```python
from build123d import *

# Parameters (mm, degrees)
BASPROSKE_W         = 5
BASPROSKE_H         = 10
TOOTHCUT_DEPTH      = 16
TEETHCUTS_COUNT     = 18
TEETHCUTS_ANGLE     = 340
BORSKE_R            = 4
BORE_DEPTH          = 50.0000508
CUT_EXTRUDE_1_DEPTH = 2.5


with BuildPart() as part:
    # BasProSke → Base-Revolve (revolve)
    with BuildSketch(Plane(origin=(0, 0, 0), x_dir=(1, 0, 0), z_dir=(0, 1, 0)), mode=Mode.PRIVATE) as base_revolve_sk:
        with Locations((2.5, 5)):
            Rectangle(BASPROSKE_W, BASPROSKE_H)
    revolve(base_revolve_sk.sketch.rotate(Axis((-10, 0, 0), (1, 0, 0)), 180), axis=Axis((-10, 0, 0), (1, 0, 0)))

    # TooCutSke → ToothCut (cut, through all)
    with BuildSketch(Plane(origin=(0, 0, 0), x_dir=(0, 0, -1), z_dir=(1, 0, 0))):
        with BuildLine():
            ThreePointArc((0.510641536, 7.732156635), (0, 7.749), (-0.510641536, 7.732156635))
            ThreePointArc((-0.510641536, 7.732156635), (-0.82619259, 8.907320741), (-1.515208602, 9.910236529))
            ThreePointArc((-1.515208602, 9.910236529), (0, 10.0254), (1.515208602, 9.910236529))
            ThreePointArc((1.515208602, 9.910236529), (0.82619259, 8.907320741), (0.510641536, 7.732156635))
        make_face()
    toothcut = extrude(amount=TOOTHCUT_DEPTH, mode=Mode.SUBTRACT)

    # TeethCuts: ToothCut ×18 about axis
    teethcuts_axis = Axis((-10, 0, 0), (1, 0, 0))
    for i in range(1, TEETHCUTS_COUNT):
        add(toothcut.rotate(teethcuts_axis, i * TEETHCUTS_ANGLE / (TEETHCUTS_COUNT - 1)), mode=Mode.SUBTRACT)

    # BorSke → Bore (cut, symmetric)
    with BuildSketch(Plane(origin=(0, 0, 0), x_dir=(0, 0, -1), z_dir=(1, 0, 0))):
        with Locations(Location((0, 0, 0), (0, 0, 180))):
            Circle(BORSKE_R)
    extrude(amount=BORE_DEPTH, both=True, mode=Mode.SUBTRACT)

    # 草图2 → 切除-拉伸1 (cut)
    with BuildSketch(Plane.ZY):
        Polygon((0.391153716, 3.478074003), (-0.822007108, -3.402102925), (-15.361721341, -0.838359014), (-14.148560516, 6.041817914), align=None)
    extrude(amount=-CUT_EXTRUDE_1_DEPTH, mode=Mode.SUBTRACT)


solid = part.part
```
Input: part model. Units: mm. Frame: model coordinates. A direction names the side the tool comes from. Round coordinates to 2 decimals unless told otherwise and drop trailing zeros. Order: outer loops, then holes, each group sorted by start corner. A loop starts at its lowest first (then second) coordinate and runs counter-clockwise, first axis right, second up. Notation, with made-up numbers: (57.25, 53) - (108.25, 53) arc R21 cw to (108.25, 91) - close; hole circle Ø3 at (51.5, 77.25). An arc over 180 degrees is marked (long way). One line per question, with ' | ' between items. Start each with the question number.
1) Ray query, probe 1 along Y at (x, z) = (1.5, 0); probe 2 along Z at (x, y) = (1.85, 6); probe 3 along Y at (x, z) = (1.25, 8.5). Return the intervals inside material, ascending.
2) Cut plane A-A, the plane y = 0. Return the cut outline in (x, z), then the cut area to 3 significant figures.
3) Contact query for a flat-ended pin moving along its axis: P1, Ø3, axis at x = 3, y = -7.5, coming from the +Z side. Output: stop coordinate, or through.
4) Set-up query: faces 4 (the cylindrical face through (2.465, 8.878, 0.813)), 5 (the cylindrical face through (2.46, -5.17, -7.3)), 6 (the cylindrical face through (2.465, -7.323, 5.084)). Return all of +Z, -Z, +X, -X, +Y, -Y with unobstructed straight access to the full face (end or side cutting, diameter ignored); none if empty.
5) Cut plane B-B, the plane z = 0. Return the cut outline in (x, y), then the cut area to 3 significant figures.
6) Cut plane C-C, the plane y = -8. Return the cut outline in (x, z).
7) Pull-direction query (Z, two-part tool) for faces 1 (the cylindrical face through (2.465, 5.366, -7.431)), 2 (the flat face through (0, 0, 5)), 3 (the flat face through (1.23, -2.61, -5.32)); classes: +Z half, -Z half, draft (parallel to the pull), parting line (faces both ways), or undercut.
Worked out:
1) probe 1: y = -7.75 to -4, 4 to 7.75 | probe 2: z = -7.74 to -5.85, -4.9 to 4.9, 5.85 to 7.74 | probe 3: y = -3.75 to -2.28, -0.82 to 0.82, 2.28 to 3.75
2) outline: (0, 4) - (5, 4) - (5, 10) - (0, 10) - close; (2.5, -10) - (5, -10) - (5, -4) - (2.5, -4) - close | area: 45.0 mm^2
3) P1: stops at z = 7.82
4) face 4: +X, -X, +Y | face 5: -Z, +X, -X | face 6: +X, -X
5) outline: (0, -7.75) - (5, -7.75) - (5, -4) - (0, -4) - close; (0, 4) - (5, 4) - (5, 7.75) - (0, 7.75) - close | area: 37.5 mm^2
6) outline: (0, -5.21) - (5, -5.21) - (5, -3.74) - (0, -3.74) - close; (0, -2.27) - (5, -2.27) - (5, -0.55) - (0, -0.55) - close; (0, 0.55) - (5, 0.55) - (5, 2.27) - (0, 2.27) - close; (0, 3.74) - (5, 3.74) - (5, 5.21) - (0, 5.21) - close
7) face 1: -Z half | face 2: draft | face 3: undercut
